from build123d import *

# Parameters (mm, degrees)
FILLET1_R     = 10
CHAMFER1_SIZE = 1


with BuildPart() as part:
    # Sketch1 → Revolve1 (revolve)
    with BuildSketch(Plane.XY, mode=Mode.PRIVATE) as revolve1_sk:
        Polygon((-137.5, 0), (137.5, 0), (137.5, 10), (-71.5, 10), (-75.5, 6), (-137.5, 6), align=None)
    revolve(revolve1_sk.sketch.rotate(Axis((-137.5, 0, 0), (1, 0, 0)), 90), axis=Axis((-137.5, 0, 0), (1, 0, 0)))

    # Fillet1
    fillet1_edges = [part.edges().sort_by_distance(p)[0] for p in [
        (137.5, 0, -10),
    ]]
    fillet(fillet1_edges, radius=FILLET1_R)

    # Chamfer1
    chamfer1_edges = [part.edges().sort_by_distance(p)[0] for p in [
        (-137.5, 0, -6),
    ]]
    chamfer(chamfer1_edges, length=CHAMFER1_SIZE)


solid = part.part
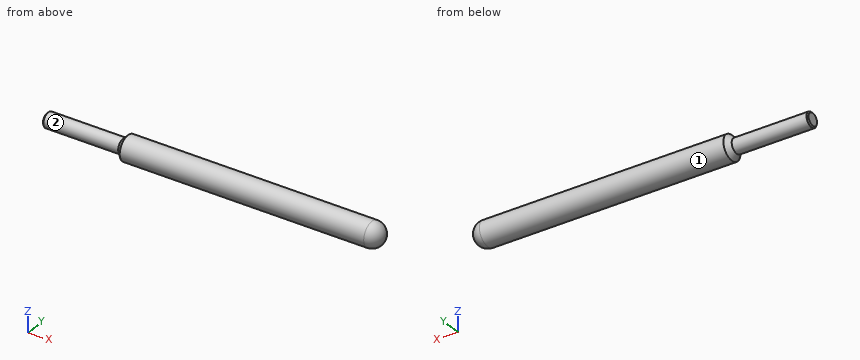
Could you check a few things on this model? Use its own coordinates, in mm. Face numbers are marked on the shaded views. A direction names the side the tool comes from. Coordinates: 2 decimals unless noted, no trailing zeros. Loops run counter-clockwise (first coordinate to the right, second up) from the corner with the lowest first, then second, coordinate; pieces in that order, holes last.
1. For the marked faces 1 and 2, which set-ups out of +Z, -Z, +X, -X, +Y, -Y let a thin tool reach every point of the face, with its end or its side?
2. For P1, Ø5, axis at x = -77, y = 1.5, coming from the +Z side; P2, Ø5, axis at x = -37.5, y = 6, coming from the +Z side; P3, Ø1, axis at x = 3, z = -3.5, coming from the +Y side; P4, Ø10, axis at y = 0, z = -2, coming from the +X side, each with a flat end and sliding along its axis, tell me the tip position at first contact or that it passes through.
3. Imagine slicing it at D-D (x = -53.5). Please give me the cut outline in (y, z), and give its area (3 significant figures).
4. I need wall thicknesses on L1, parallel to Z at x = -11.5, y = -0.5; L2, parallel to Y at x = 19, z = -8; L3, parallel to X at y = 8.75, z = 2. Which ranges of each line are inside material? Lowest first, please.
5. Imagine slicing it at C-C (x = -82). Please give me the cut outline in (y, z).
6. Imagine slicing it at A-A (y = 0). Please give me the cut outline in (x, z), and give its area (3 significant figures).
Computed values:
1. face 1: +X, -X
1. face 2: -X
2. P1: stops at z = 6.88
2. P2: stops at z = 9.37
2. P3: stops at y = 9.54
2. P4: stops at x = 137.5
3. outline: circle Ø20 at (0, 0)
3. area: 314 mm2
4. L1: z = -9.99 to 9.99
4. L2: y = -6 to 6
4. L3: x = -72.52 to 131.91
5. outline: circle Ø12 at (0, 0)
6. outline: (-137.5, -5) - (-136.5, -6) - (-75.5, -6) - (-71.5, -10) - (127.5, -10) arc R10 ccw to (127.5, 10) - (-71.5, 10) - (-75.5, 6) - (-136.5, 6) - (-137.5, 5) - close
6. area: 4,940 mm2
